from build123d import *

# Parameters (mm, degrees)
SKETCH_R     = 4.25
PAD_DEPTH    = 10
SKETCH001_W  = 16
SKETCH001_H  = 16
POCKET_DEPTH = 5
FILLET_R     = 7


with BuildPart() as part:
    # Sketch → Pad (new body)
    with BuildSketch(Plane.XY):
        with BuildLine():
            ThreePointArc((0, -57.5), (57.5, 0), (0, 57.5))
            Line((0, 64.565858), (0, 57.5))
            Line((-7.5, 64.565858), (0, 64.565858))
            Line((-7.5, 79.565858), (-7.5, 64.565858))
            Line((7.5, 79.565858), (-7.5, 79.565858))
            Line((7.5, 64.565858), (7.5, 79.565858))
            ThreePointArc((7, -64.621978), (64.999513, -0.25157), (7.5, 64.565858))
            Line((7, -64.621978), (7, -79.621978))
            Line((7, -79.621978), (0, -79.621978))
            Line((0, -79.621978), (0, -57.5))
        make_face()
        with Locations((0, 72.065858)):
            Circle(SKETCH_R, mode=Mode.SUBTRACT)
    extrude(amount=PAD_DEPTH)

    # Sketch001 (on Face13 of Pad) → Pocket (cut)
    with BuildSketch(Plane.XY.offset(10)):
        with Locations((-0.5, 72.5)):
            Rectangle(SKETCH001_W, SKETCH001_H)
    extrude(amount=-POCKET_DEPTH, mode=Mode.SUBTRACT)

    # Fillet
    fillet_edges = [part.edges().sort_by_distance(p)[0] for p in [
        (-7.5, 64.565858, 2.5),
        (-7.5, 79.565858, 2.5),
    ]]
    fillet(fillet_edges, radius=FILLET_R)


solid = part.part
Could you check a few things on this model? Use its own coordinates, in mm. A direction names the side the tool comes from. Give positions to 0.01 mm unless a question says otherwise; leave off trailing zeros. Write each loop counter-clockwise with the first axis right and the second up, starting at its lowest first coordinate (ties: lowest second). Pieces come first, ordered by that corner, then holes. Notation, with made-up numbers: (-5, -30.75) -> (40, -30.75) arc R35 ccw to (40, 8.25) -> close; hole circle Ø5 at (29, -31.75). An arc over 180 degrees is marked (long way). Write each question's results on one line, items separated by ' | '. Start each with the question number.
Q1. Suppose I cut it at A-A, the plane x = 31.5. List the corners of the cut face in (y, z) for me, and give its area (3 significant figures).
Q2. Suppose I cut it at D-D, the plane x = 46. List the corners of the cut face in (y, z) for me.
Q3. We'd pull the mould along X, two halves only. Please class faces 1 (the face through (1.961, 68.295, 2.465)), 2 (the face through (-5.395, 66.562, 2.535)), 3 (the face through (7.5, 72, 2)), 4 (the face through (57, -13, 10)): +X half, -X half, draft (parallel to the pull), parting line (faces both ways), or undercut.
Q4. Suppose I cut it at B-B, the plane z = 7.25. List the corners of the cut face in (x, y) for me.
Q5. I'm going to push flat-ended pins straight in: pin 1 Ø3 at (y, z) = (-66, 3.5) entering from -X; pin 2 Ø3 at (x, z) = (36.5, 4.5) entering from -Y; pin 3 Ø6 at (x, z) = (41, 2) entering from -Y. Where does each tip first touch, or does it pass through?
Q6. Suppose I cut it at C-C, the plane y = 0. List the corners of the cut face in (x, z) for me, and give its area (3 significant figures).
Q7. I need wall thicknesses on probe 1 along Y at (x, z) = (13.5, 8.5); probe 2 along Y at (x, z) = (8, 1.75); probe 3 along X at (y, z) = (-70.5, 2). Which ranges of each line are inside material? Lowest first, please.
Q8. Which directions (+Z, -Z, +X, -X, +Y, -Y) give clear straight access to the entire face, cutting with the end or side of a thin tool? Please do faces 5 (the face through (57.486, -1.264, 4.93)), 6 (the face through (0, 61, 5)), 7 (the face through (7, -72, 5)).
Outcome:
1) outline: (-56.86, 0) -> (-48.1, 0) -> (-48.1, 10) -> (-56.86, 10) -> close; (48.1, 0) -> (56.86, 0) -> (56.86, 10) -> (48.1, 10) -> close | area: 175 mm2
2) outline: (-45.92, 0) -> (-34.5, 0) -> (-34.5, 10) -> (-45.92, 10) -> close; (34.5, 0) -> (45.92, 0) -> (45.92, 10) -> (34.5, 10) -> close
3) face 1: undercut | face 2: -X half | face 3: +X half | face 4: draft
4) outline: (0, -79.62) -> (7, -79.62) -> (7, -64.62) arc R65 ccw to (7.5, 64.57) -> (7.5, 64.5) -> (0, 64.5) -> (0, 57.5) arc R57.5 cw to (0, -57.5) -> close
5) pin 1: x = 0 | pin 2: y = -54.77 | pin 3: y = -52.74
6) outline: (57.5, 0) -> (65, 0) -> (65, 10) -> (57.5, 10) -> close | area: 75.0 mm2
7) probe 1: -63.58 to -55.89, 55.89 to 63.58 | probe 2: -64.51 to -56.94, 56.94 to 64.51 | probe 3: 0 to 7
8) face 5: +Z, -Z, -X | face 6: +Z, -Z, -X, -Y | face 7: +Z, -Z, +X, -Y
